For this review, take the finished solid that the model builds, in its own axes (mm). Face numbers are marked on the shaded views. A direction names the side the tool comes from. Round coordinates to 2 decimals unless told otherwise and drop trailing zeros. Write each loop counter-clockwise with the first axis right and the second up, starting at its lowest first coordinate (ties: lowest second). Pieces come first, ordered by that corner, then holes.
from build123d import *

# Parameters (mm, degrees)
F0_W        = 914.4
F0_H        = 304.8
F1_DEPTH    = 88.9
F2_W        = 76.2
F2_H        = 304.8
F3_DEPTH    = 304.8
F5_DEPTH    = 876.301
F6_T1_DEPTH = 342.9


# Not quite as in the source:
# - a fillet or chamfer that OpenCascade refuses, or shapes differently, is made with other operations: its cross-section is extruded or revolved along the edge and cut away or added


with BuildPart() as f1:
    # F0 (on Top) → F1 (new body)
    with BuildSketch(Plane.XY):
        Rectangle(F0_W, F0_H)
    extrude(amount=F1_DEPTH)

    # F2 (on face) → F3 (join)
    with BuildSketch(Plane.XY.offset(88.9)):
        with Locations((-381, 0)):
            Rectangle(F2_W, F2_H)
        with Locations((381, 0)):
            Rectangle(F2_W, F2_H)
    extrude(amount=F3_DEPTH)

    # F4 (on face) → F5 (cut, through all)
    with BuildSketch(Plane.YZ.offset(419.1)):
        Polygon((76.2, 292.1), (76.2, 393.7), (-152.4, 393.7), (-152.4, 88.9), align=None)
        Polygon((152.4, 88.9), (152.4, 257.8811658996), (-37.703811637, 88.9), align=None)
    extrude(amount=-F5_DEPTH, mode=Mode.SUBTRACT)

    # F6: fillet of radius 50.8 on 4 edges, made by hand

    # F6_s2 → F6_t1 (cut)
    with BuildSketch(Plane.XY.offset(-127)):
        with BuildLine():
            ThreePointArc((-457.2, -101.6), (-442.3210244843, -137.5210244843), (-406.4, -152.4))
            Line((-406.4, -152.4), (-457.2, -152.4))
            Line((-457.2, -152.4), (-457.2, -101.6))
        make_face()
        with BuildLine():
            ThreePointArc((457.2, -101.6), (442.3210244843, -137.5210244843), (406.4, -152.4))
            Line((406.4, -152.4), (457.2, -152.4))
            Line((457.2, -152.4), (457.2, -101.6))
        make_face()
        with BuildLine():
            ThreePointArc((457.2, 101.6), (442.3210244843, 137.5210244843), (406.4, 152.4))
            Line((406.4, 152.4), (457.2, 152.4))
            Line((457.2, 152.4), (457.2, 101.6))
        make_face()
        with BuildLine():
            ThreePointArc((-457.2, 101.6), (-442.3210244843, 137.5210244843), (-406.4, 152.4))
            Line((-406.4, 152.4), (-457.2, 152.4))
            Line((-457.2, 152.4), (-457.2, 101.6))
        make_face()
    extrude(amount=F6_T1_DEPTH, mode=Mode.SUBTRACT)


solid = f1.part
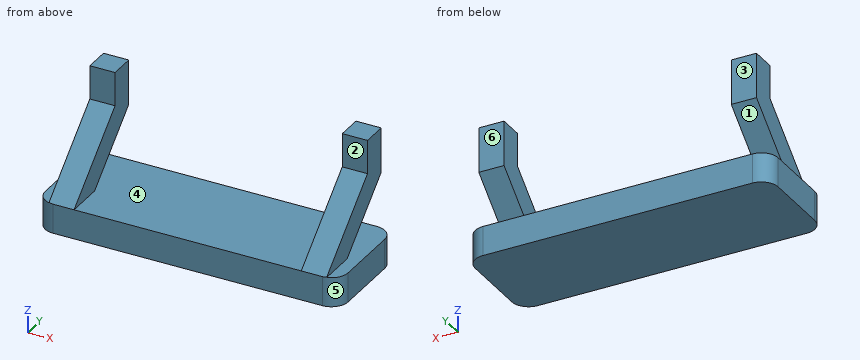
(1) We need section B-B, the plane y = 91. Give the boundary of the cut face in (x, z).
Geometry check:
outline: (-457.2, 0) - (457.2, 0) - (457.2, 88.9) - (-457.2, 88.9) - close; (-419.1, 203.3) - (-342.9, 203.3) - (-342.9, 393.7) - (-419.1, 393.7) - close; (342.9, 203.3) - (419.1, 203.3) - (419.1, 393.7) - (342.9, 393.7) - close
(2) Mouldability with a two-part tool opening along X and no side actions: class the marked faces 4, 5 and 6 as pulls with the +X half, pulls with the -X half, needs draft (parallel to the pull), parting line crosses it, or undercut.
Geometry check:
face 4: undercut
face 5: pulls with the +X half
face 6: needs draft
(3) For line 1 along X through (y, z) = (-76.5, 114); line 2 along Z through (x, y) = (173, -71.5); line 3 along Y through (x, z) = (-347, 339.5), list the stretches that pass through material, from the lowest coordinate up.
Geometry check:
line 1: x = -419.1 to -342.9, 342.9 to 419.1
line 2: z = 0 to 88.9
line 3: y = 76.2 to 152.4
(4) For the marked faces 1, 2 and 3, list the 3-axis set-ups (+Z, -Z, +X, -X, +Y, -Y) from which the entire face can be reached by the end or side of a thin tool; tool diameter is ignored.
Geometry check:
face 1: +X, -X, +Y
face 2: +Z, +X, -X, -Y
face 3: +Z, -Z, +X, -X, +Y
(5) We need section A-A, the plane z = 333.5. Give the boundary of the cut face in (x, y), and give its area (3 significant figures).
Geometry check:
outline: (-419.1, 76.2) - (-342.9, 76.2) - (-342.9, 152.4) - (-419.1, 152.4) - close; (342.9, 76.2) - (419.1, 76.2) - (419.1, 152.4) - (342.9, 152.4) - close
area: 11,600 mm2
(6) We need section D-D, the plane y = -78. Give the boundary of the cut face in (x, z), and give its area (3 significant figures).
Geometry check:
outline: (-457.2, 0) - (457.2, 0) - (457.2, 88.9) - (419.1, 88.9) - (419.1, 155.03) - (342.9, 155.03) - (342.9, 88.9) - (-342.9, 88.9) - (-342.9, 155.03) - (-419.1, 155.03) - (-419.1, 88.9) - (-457.2, 88.9) - close
area: 91,400 mm2
(7) For pin 1 Ø23 at (x, z) = (-383, 350) entering from -Y; pin 2 Ø4 at (x, y) = (264, -67) entering from +Z, all flat-tipped, find the tip position at first contact; note any pin that passes through.
Geometry check:
pin 1: stops at y = 76.2
pin 2: stops at z = 88.9
(8) We need section C-C, the plane x = -390. Give the boundary of the cut face in (y, z), and give its area (3 significant figures).
Geometry check:
outline: (-152.4, 0) - (152.4, 0) - (152.4, 88.9) - (-37.7, 88.9) - (152.4, 257.88) - (152.4, 393.7) - (76.2, 393.7) - (76.2, 292.1) - (-152.4, 88.9) - close
area: 57,500 mm2
